from build123d import *

# Parameters (mm, degrees)
F0_R     = 22.5603447523
F0_R_2   = 21.5516802716
F0_R_3   = 9.418040514
F0_R_4   = 16.7395174503
F0_R_5   = 11.6092445083
F0_R_6   = 16.8526987349
F1_DEPTH = 4


# Not quite as in the source:
# - ends of sketch curves that miss each other by under 0.0002 mm in the source are joined


with BuildPart() as f1:
    # F0 (on Front) → F1 (new body)
    with BuildSketch(Plane.XZ):
        with BuildLine():
            Line((78.8341670899, -6.8383235484), (114.8409428481, -6.8383235484))
            Line((114.8409428481, -6.8383235484), (114.8409428481, 0.6616764516))
            Line((114.8409428481, 0.6616764516), (128.8409428481, 0.6616764516))
            add(Edge.make_bspline(
                [(124.9033857451, 130.1616764516), (127.8407562373, 89.5517987134), (128.7514642032, 44.6895821219), (128.8409428481, 0.6616764516)],
                knots=[0.2778483476, 0.2778483476, 0.2778483476, 0.2778483476, 0.4880499366, 0.4880499366, 0.4880499366, 0.4880499366], degree=3))
            Line((124.9033857451, 130.1616764516), (110.9033857451, 130.1616764516))
            Line((110.9033857451, 130.1616764516), (110.9033857451, 137.6616764516))
            Line((110.9033857451, 137.6616764516), (77.7980855424, 137.6616764516))
            Line((77.7980855424, 137.6616764516), (77.7980855424, 130.1616764516))
            Line((77.7980855424, 130.1616764516), (63.7980855424, 130.1616764516))
            add(Edge.make_bspline(
                [(63.7980855424, 130.1616764516), (64.3462926476, 86.9798084925), (64.7350115683, 43.8051528282), (64.8341670899, 0.6616764516)],
                knots=[0.2404841481, 0.2404841481, 0.2404841481, 0.2404841481, 0.4857851385, 0.4857851385, 0.4857851385, 0.4857851385], degree=3))
            Line((64.8341670899, 0.6616764516), (78.8341670899, 0.6616764516))
            Line((78.8341670899, 0.6616764516), (78.8341670899, -6.8383235484))
        make_face()
        with Locations((93.8518792391, 71.5714693069)):
            Circle(F0_R, mode=Mode.SUBTRACT)
        with Locations((95.6616252661, 22.0235623419)):
            Circle(F0_R_2, mode=Mode.SUBTRACT)
        with Locations((95.5336689949, 117.9889589548)):
            Circle(F0_R_3, mode=Mode.SUBTRACT)
        with BuildLine():
            Line((110.9033857451, 145.1616764516), (123.7062231815, 145.1616764516))
            add(Edge.make_bspline(
                [(99.8484624624, 257.1616764516), (112.2986005896, 232.646487185), (119.5620823416, 192.4052892247), (123.7062231815, 145.1616764516)],
                knots=[0, 0, 0, 0, 0.2516076621, 0.2516076621, 0.2516076621, 0.2516076621], degree=3))
            Line((99.8484624624, 257.1616764516), (61.8484624624, 257.1616764516))
            add(Edge.make_bspline(
                [(61.8484624624, 257.1616764516), (62.5273104324, 217.3359288807), (63.1789559316, 177.4963243829), (63.701293151, 137.6616764516)],
                knots=[0, 0, 0, 0, 0.2262826567, 0.2262826567, 0.2262826567, 0.2262826567], degree=3))
            Line((63.701293151, 137.6616764516), (77.7980855424, 137.6616764516))
            Line((77.7980855424, 137.6616764516), (110.9033857451, 137.6616764516))
            Line((110.9033857451, 137.6616764516), (110.9033857451, 145.1616764516))
        make_face()
        with Locations((92.5064459443, 163.3973568678)):
            Circle(F0_R_4, mode=Mode.SUBTRACT)
        with Locations((83.761125803, 238.4053170681)):
            Circle(F0_R_5, mode=Mode.SUBTRACT)
        with Locations((88.47014606, 203.7603855133)):
            Circle(F0_R_6, mode=Mode.SUBTRACT)
        with BuildLine():
            Line((114.8409428481, -14.3383235484), (114.8409428481, -6.8383235484))
            Line((114.8409428481, -6.8383235484), (78.8341670899, -6.8383235484))
            Line((78.8341670899, -6.8383235484), (78.8341670899, -14.3383235484))
            Line((78.8341670899, -14.3383235484), (64.8568045286, -14.3383235484))
            add(Edge.make_bspline(
                [(64.8568045286, -14.3383235484), (64.8876732357, -57.5094122228), (64.6230490688, -100.6520537776), (64.0989954927, -143.8383235484)],
                knots=[0.51421607, 0.51421607, 0.51421607, 0.51421607, 0.7597151822, 0.7597151822, 0.7597151822, 0.7597151822], degree=3))
            Line((64.0989954927, -143.8383235484), (77.7980855424, -143.8383235484))
            Line((77.7980855424, -143.8383235484), (77.7980855424, -151.3383235484))
            Line((77.7980855424, -151.3383235484), (77.7980855424, -158.8383235484))
            Line((77.7980855424, -158.8383235484), (63.9066232608, -158.8383235484))
            add(Edge.make_bspline(
                [(63.9066232608, -158.8383235484), (63.4029478239, -196.117508426), (62.7091678723, -233.4354001086), (61.8484624624, -270.8383235484)],
                knots=[0.7881349295, 0.7881349295, 0.7881349295, 0.7881349295, 1, 1, 1, 1], degree=3))
            Line((61.8484624624, -270.8383235484), (99.8484624624, -270.8383235484))
            add(Edge.make_bspline(
                [(123.2627847104, -158.8383235484), (119.0509791243, -202.5082607649), (111.8659348538, -240.9997580131), (99.8484624624, -270.8383235484)],
                knots=[0.7571361778, 0.7571361778, 0.7571361778, 0.7571361778, 1, 1, 1, 1], degree=3))
            Line((123.2627847104, -158.8383235484), (110.9033857451, -158.8383235484))
            Line((110.9033857451, -158.8383235484), (110.9033857451, -151.3383235484))
            Line((110.9033857451, -151.3383235484), (110.9033857451, -143.8383235484))
            Line((110.9033857451, -143.8383235484), (124.5795751588, -143.8383235484))
            add(Edge.make_bspline(
                [(128.8408993214, -14.3383234592), (128.7479516437, -59.6820922187), (127.7738982193, -103.6829779906), (124.5795751588, -143.8383235484)],
                knots=[0.5119840968, 0.5119840968, 0.5119840968, 0.5119840968, 0.7296879862, 0.7296879862, 0.7296879862, 0.7296879862], degree=3))
            Line((128.8408993214, -14.3383234592), (114.8409428481, -14.3383235484))
        make_face()
        with Locations((83.761125803, -252.081964165)):
            Circle(F0_R_5, mode=Mode.SUBTRACT)
        with Locations((88.47014606, -217.4370326102)):
            Circle(F0_R_6, mode=Mode.SUBTRACT)
        with Locations((92.5064459443, -177.0740039647)):
            Circle(F0_R_4, mode=Mode.SUBTRACT)
        with Locations((93.8518792391, -85.2481164038)):
            Circle(F0_R, mode=Mode.SUBTRACT)
        with Locations((95.5336689949, -131.6656060517)):
            Circle(F0_R_3, mode=Mode.SUBTRACT)
        with Locations((95.6616252661, -35.7002094388)):
            Circle(F0_R_2, mode=Mode.SUBTRACT)
    extrude(amount=F1_DEPTH)


solid = f1.part
Build history of the part. All positions in model axes, mm. Round coordinates to 2 decimals unless told otherwise and drop trailing zeros. One line per item, written item: value. Start each with the question number.
Q1. Probe line 1 along Z through (x, y) = (66, -0.35); line 2 along X through (y, z) = (-1.9, 66); line 3 along X through (y, z) = (-1, 41.5). List the from-to ranges inside material, lowest first.
Q2. Two-plate mould, pull along X, no slides. Class faces 1 (the face through (116.218, -1.972, 28.497)), 2 (the face through (95, -4, -3)), 3 (the face through (115.57, -1.97, -43.95)): released by +X, released by -X, zero draft, split by the parting line, or undercut.
Q3. Drop a flat-ended pin along its axis: pin 1 Ø1.2 at (y, z) = (-2.5, -5.5) entering from -X. Give the stop position or say it passes through.
Q4. Cut at A-A on y = -3.05. Count the separate pieces of the cut face and the enclosed holes in it, plus the area to 3 significant figures.
Computed:
1. line 1: -270.84 to -158.84, -143.84 to -14.34, 0.66 to 130.16, 137.66 to 257.16
1. line 2: 64.48 to 71.99, 115.71 to 127.96
1. line 3: 64.66 to 86.43, 104.89 to 128.49
2. face 1: undercut
2. face 2: zero draft
2. face 3: undercut
3. pin 1: x = 78.83
4. separate pieces: 1
4. enclosed holes: 12
4. area: 18,500 mm²
